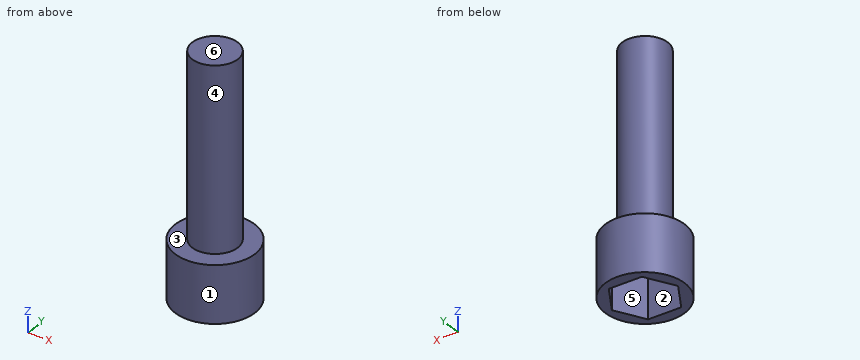
from build123d import *

# Parameters (mm, degrees)
CROQUIS1_R              = 1.75
SALIENTE_EXTRUIR1_DEPTH = 2.5
CROQUIS2_R              = 1
SALIENTE_EXTRUIR2_DEPTH = 8
CORTAR_EXTRUIR1_DEPTH   = 1.75


with BuildPart() as part:
    # Croquis1 → Saliente-Extruir1 (new body)
    with BuildSketch(Plane.XY):
        Circle(CROQUIS1_R)
    extrude(amount=SALIENTE_EXTRUIR1_DEPTH)

    # Croquis2 → Saliente-Extruir2 (add)
    with BuildSketch(Plane.XY.offset(2.5)):
        Circle(CROQUIS2_R)
    extrude(amount=SALIENTE_EXTRUIR2_DEPTH)

    # Croquis3 → Cortar-Extruir1 (cut)
    with BuildSketch(Plane(origin=(0, 0, 0), x_dir=(-1, 0, 0), z_dir=(0, 0, -1))):
        Polygon((1.443375673, 0), (0.721687836, 1.25), (-0.721687836, 1.25), (-1.443375673, 0), (-0.721687836, -1.25), (0.721687836, -1.25), align=None)
    extrude(amount=-CORTAR_EXTRUIR1_DEPTH, mode=Mode.SUBTRACT)


solid = part.part
Source: CAD feature listing. Evaluate the final solid. Frame: model axes, mm. Face numbers are marked on the shaded views. A direction names the side the tool comes from. Round coordinates to 2 decimals unless told otherwise and drop trailing zeros. Loops run counter-clockwise (first coordinate to the right, second up) from the corner with the lowest first, then second, coordinate; pieces in that order, holes last. Notation, with made-up numbers: (72, -23.75) - (100, -23.75) arc R18 ccw to (100, -11.75) - close; hole circle Ø9 at (37, 38). An arc over 180 degrees is marked (long way). Write item = value, one per line. Start each with the question number.
Item 1: Reachability of the marked faces 4, 5 and 6 from +Z, -Z, +X, -X, +Y, -Y: full face, straight path, thin tool, end or side. Return the list, or none.
Item 2: Section query B-B on y = 0.4. Output: boundary loops of the cut face in (x, z).
Item 3: Material intervals for line 1 (Z direction, x = 0.25, y = 0.45); line 2 (Z direction, x = -0.55, y = -1); line 3 (Y direction, x = 1.2, z = 1.25), sorted ascending.
Item 4: Section query D-D on x = 1.55. Output: boundary loops of the cut face in (y, z).
Item 5: Section query C-C on z = 6.75. Output: boundary loops of the cut face in (x, y), plus the area to 3 significant figures.
Item 6: Mould query, pull axis Y, two halves, no side actions, for the marked faces 1, 2 and 3. Classes: released by +Y, released by -Y, zero draft, split by the parting line, or undercut.
Item 7: Section query A-A on x = 0. Output: boundary loops of the cut face in (y, z), plus the area to 3 significant figures.
Results list:
q1.face_4 = +Z
q1.face_5 = -Z
q1.face_6 = +Z, +X, -X, +Y, -Y
q2.outline = (-1.7, 0) - (-1.21, 0) - (-1.21, 1.75) - (1.21, 1.75) - (1.21, 0) - (1.7, 0) - (1.7, 2.5) - (0.92, 2.5) - (0.92, 10.5) - (-0.92, 10.5) - (-0.92, 2.5) - (-1.7, 2.5) - close
q3.line_1 = 1.75 to 10.5
q3.line_2 = 1.75 to 2.5
q3.line_3 = -1.27 to -0.42, 0.42 to 1.27
q4.outline = (-0.81, 0) - (0.81, 0) - (0.81, 2.5) - (-0.81, 2.5) - close
q5.outline = circle Ø2 at (0, 0)
q5.area = 3.14 mm²
q6.face_1 = split by the parting line
q6.face_2 = undercut
q6.face_3 = zero draft
q7.outline = (-1.75, 0) - (-1.25, 0) - (-1.25, 1.75) - (1.25, 1.75) - (1.25, 0) - (1.75, 0) - (1.75, 2.5) - (1, 2.5) - (1, 10.5) - (-1, 10.5) - (-1, 2.5) - (-1.75, 2.5) - close
q7.area = 20.4 mm²
